Answer from the drawing. Dimensions are ordinates in mm from the lowest x, y and z of the part. Coordinates: 2 decimals unless noted, no trailing zeros. Write each loop counter-clockwise with the first axis right and the second up, starting at its lowest first coordinate (ties: lowest second). Pieces come first, ordered by that corner, then holes.
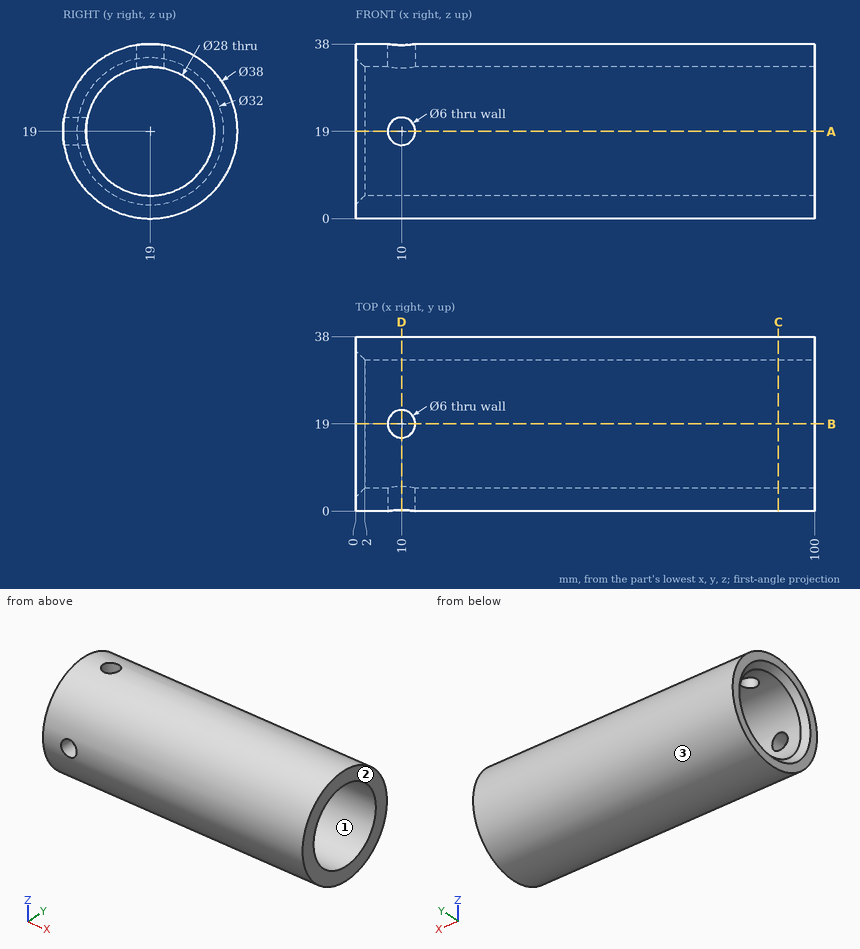
(1) Section D-D, the plane x = 10 is taken. Write down the section's boundary in (y, z), plus the area to 3 significant figures.
(2) For a pull along Y with two mould halves and no side action, classify the marked faces 1, 2 and 3 as pulls with the +Y half, pulls with the -Y half, needs draft (parallel to the pull), parting line crosses it, or undercut.
(3) Section C-C, the plane x = 92 is taken. Write down the section's boundary in (y, z), plus the area to 3 significant figures.
(4) Find the intervals of material crossed by probe 1 along Z at (x, y) = (62, 19); probe 2 along Y at (x, z) = (24, 24.5); probe 3 along Z at (x, y) = (65.5, 17), in increasing order.
(5) Each of these flat-tipped pins is pushed along its axis until it touches: pin 1 (1.5 mm diameter, centred on x = 24, z = 4, fed in from -Y); pin 2 (3 mm diameter, centred on x = 10.5, z = 21.5, fed in from +Y); pin 3 (1.5 mm diameter, centred on x = 38.5, z = 13, fed in from -Y). Where does it stop, or does it pass through?
(6) Section A-A, the plane z = 19 is taken. Write down the section's boundary in (x, y), plus the area to 3 significant figures.
(7) Section B-B, the plane y = 19 is taken. Write down the section's boundary in (x, z), plus the area to 3 significant figures.
Solution:
1. outline: (0.24, 16) arc R19 ccw (long way) to (22, 37.76) - (22, 32.67) arc R14 cw (long way) to (5.33, 16) - close; (0.24, 22) - (5.33, 22) arc R14 cw to (16, 32.67) - (16, 37.76) arc R19 ccw to start
1. area: 458 mm2
2. face 1: undercut
2. face 2: needs draft
2. face 3: parting line crosses it
3. outline: circle Ø38 at (19, 19); hole circle Ø28 at (19, 19)
3. area: 518 mm2
4. probe 1: z = 0 to 5, 33 to 38
4. probe 2: y = 0.81 to 6.13, 31.87 to 37.19
4. probe 3: z = 0.11 to 5.14, 32.86 to 37.89
5. pin 1: stops at y = 6.43
5. pin 2: stops at y = 37.97
5. pin 3: stops at y = 0.74
6. outline: (0, 0) - (7, 0) - (7, 5) - (2, 5) - (0, 3) - close; (0, 35) - (2, 33) - (100, 33) - (100, 38) - (0, 38) - close; (13, 0) - (100, 0) - (100, 5) - (13, 5) - close
6. area: 966 mm2
7. outline: (0, 0) - (100, 0) - (100, 5) - (2, 5) - (0, 3) - close; (0, 35) - (2, 33) - (7, 33) - (7, 38) - (0, 38) - close; (13, 33) - (100, 33) - (100, 38) - (13, 38) - close
7. area: 966 mm2
